```python
from build123d import *

# Parameters (mm, degrees)
F2_SIZE  = 1.016
F3_R     = 5.6515
F4_DEPTH = 25.4
F5_SIZE  = 0.254


with BuildPart() as f1:
    # F0 (on Front) → F1 (revolve)
    with BuildSketch(Plane.XZ):
        Polygon((10.287, 9.5504), (10.287, 0), (13.5128, 0), (13.5128, 12.7), (0, 12.7), (0, 9.5504), align=None)
    revolve(axis=Axis((0, 0, 6.35), (0, 0, 1)))

    # F2
    f2_edges = [f1.edges().sort_by_distance(p)[0] for p in [
        (-13.5128, 0, 12.7),
        (-13.5128, 0, 0),
    ]]
    chamfer(f2_edges, length=F2_SIZE)

    # F3 (on face) → F4 (cut)
    with BuildSketch(Plane.XY.offset(12.7)):
        Circle(F3_R)
    extrude(amount=-F4_DEPTH, mode=Mode.SUBTRACT)

    # F5
    f5_edges = [f1.edges().sort_by_distance(p)[0] for p in [
        (-5.6515, 0, 12.7),
        (-5.6515, 0, 9.5504),
        (-10.287, 0, 0),
    ]]
    chamfer(f5_edges, length=F5_SIZE)


solid = f1.part
```
Geometry: final body of the model. Coordinates: model frame, mm. A direction names the side the tool comes from. Coordinates: 2 decimals unless noted, no trailing zeros. Order: outer loops, then holes, each group sorted by start corner. A loop starts at its lowest first (then second) coordinate and runs counter-clockwise, first axis right, second up. Notation, with made-up numbers: (-14, -7.75) -> (19, -7.75) arc R16 cw to (19, 12.25) -> close; hole circle Ø7 at (45, 30). An arc over 180 degrees is marked (long way). Write each question's results on one line, items separated by ' | '. Start each with the question number.
1) First-contact query: pin 1 (4 mm diameter, centred on y = -10.5, z = 4.5, fed in from -X); pin 2 (3 mm diameter, centred on y = -5, z = 9.5, fed in from -X); pin 3 (1.5 mm diameter, centred on x = 2.5, z = 4, fed in from -Y). Flat tips, straight axial feed; report the tip coordinate or a pass-through.
2) Cut plane C-C, the plane z = 2.5. Output: boundary loops of the cut face in (x, y), and give its area (3 significant figures).
3) Material intervals for line 1 along Y through (x, z) = (0, 11.35); line 2 along Y through (x, z) = (0, 4.5); line 3 along X through (y, z) = (-7.5, 4.75), sorted ascending.
4) Set-up query: faces 1 (the cylindrical face through (-1.34, 10.2, 4.84)), 2 (the cylindrical face through (5.39, 1.7, 11.14)). Return all of +Z, -Z, +X, -X, +Y, -Y with unobstructed straight access to the full face (end or side cutting, diameter ignored); none if empty.
5) Cut plane A-A, the plane y = 0. Output: boundary loops of the cut face in (x, z).
6) Mould query, pull axis Y, two halves, no side actions, for faces 3 (the flat face through (5.4, 3, 12.7)), 4 (the flat face through (-4.4, -4.4, 9.55)), 5 (the cylindrical face through (-10.723, -8.222, 6.425)). Classes: released by +Y, released by -Y, zero draft, split by the parting line, or undercut.
Checks:
1) pin 1: x = -10.5 | pin 2: x = -13.05 | pin 3: y = -13.4
2) outline: circle Ø27.03 at (0, 0); hole circle Ø20.57 at (0, 0) | area: 241 mm^2
3) line 1: -13.51 to -5.65, 5.65 to 13.51 | line 2: -13.51 to -10.29, 10.29 to 13.51 | line 3: -11.24 to -7.04, 7.04 to 11.24
4) face 1: -Z | face 2: +Z, -Z
5) outline: (-13.51, 1.02) -> (-12.5, 0) -> (-10.54, 0) -> (-10.29, 0.25) -> (-10.29, 9.55) -> (-5.91, 9.55) -> (-5.65, 9.8) -> (-5.65, 12.45) -> (-5.91, 12.7) -> (-12.5, 12.7) -> (-13.51, 11.68) -> close; (5.65, 9.8) -> (5.91, 9.55) -> (10.29, 9.55) -> (10.29, 0.25) -> (10.54, 0) -> (12.5, 0) -> (13.51, 1.02) -> (13.51, 11.68) -> (12.5, 12.7) -> (5.91, 12.7) -> (5.65, 12.45) -> close
6) face 3: zero draft | face 4: undercut | face 5: split by the parting line
